Geometry: see drawing. Coordinates: mm, zero at the bounding-box minimum. Round coordinates to 2 decimals unless told otherwise and drop trailing zeros. Loops run counter-clockwise (first coordinate to the right, second up) from the corner with the lowest first, then second, coordinate; pieces in that order, holes last. Notation, with made-up numbers: M 4,46 L 52,46 A27 cw 52,66 Z; hole C -4,-11 d3. An arc over 180 degrees is marked long. Answer as a JSON object with one key per item and string values.
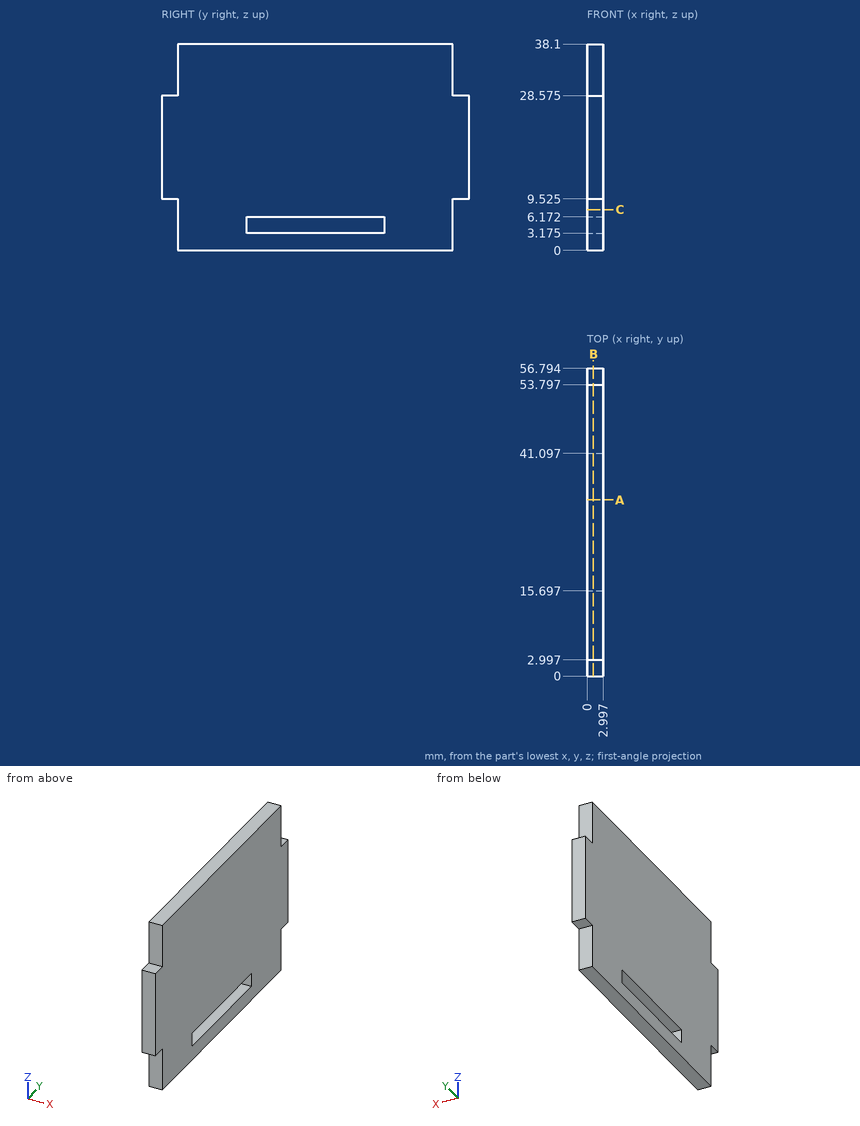
1) Section query A-A (y = 32.5). Return the cut outline in (x, z) (1 decimal).
Results:
{"outline": "M 0,0 L 3,0 L 3,3.2 L 0,3.2 Z; M 0,6.2 L 3,6.2 L 3,38.1 L 0,38.1 Z"}
2) Section query C-C (z = 7.5). Return the cut outline in (x, y).
Results:
{"outline": "M 0,3 L 3,3 L 3,53.8 L 0,53.8 Z"}
3) Ray query, line 1 (Z direction, x = 2.6, y = 17) (1 decimal); line 2 (Y direction, x = 0.35, z = 4); line 3 (Y direction, x = 2.1, z = 2). Return the intervals inside material, ascending.
Results:
{"line 1": "0 to 3.2, 6.2 to 38.1", "line 2": "3 to 15.7, 41.1 to 53.8", "line 3": "3 to 53.8"}
4) Pin query (flat end, axial travel): P1, Ø1.5, axis at x = 2, z = 5.5, coming from the -Y side; P2, Ø4, axis at y = 29.5, z = 31.5, coming from the -X side; P3, Ø1.5, axis at x = 1.5, y = 1, coming from the +Z side (3 decimals). Return the tip coordinate at first contact, or that it passes through.
Results:
{"P1": "y = 3", "P2": "x = 0", "P3": "z = 28.575"}
5) Section query B-B (x = 1.15). Return the cut outline in (y, z) (1 decimal).
Results:
{"outline": "M 0,9.5 L 3,9.5 L 3,0 L 53.8,0 L 53.8,9.5 L 56.8,9.5 L 56.8,28.6 L 53.8,28.6 L 53.8,38.1 L 3,38.1 L 3,28.6 L 0,28.6 Z; hole M 15.7,3.2 L 41.1,3.2 L 41.1,6.2 L 15.7,6.2 Z"}
